Part model, mm, in its own coordinate system. Face numbers are marked on the shaded views. A direction names the side the tool comes from. Coordinates: 2 decimals unless noted, no trailing zeros. Loops run counter-clockwise (first coordinate to the right, second up) from the corner with the lowest first, then second, coordinate; pieces in that order, holes last. Notation, with made-up numbers: (16.25, 32.25) - (38.25, 32.25) arc R12 ccw to (38.25, 38.25) - close; hole circle Ø5 at (-1.75, 25.25). An arc over 180 degrees is marked (long way). Answer as CSV lines item,"result".
from build123d import *

# Parameters (mm, degrees)
SKETCH_1_W          = 4
SKETCH_1_H          = 5.1
EXTRUDE_1_DEPTH     = 5
SKETCH_2_R          = 3
CUT_EXTRUDE_1_DEPTH = 10
SKETCH_3_R          = 7
SKETCH_3_R_2        = 4
EXTRUDE_2_DEPTH     = 4
CHAMFER_1_SIZE      = 0.5
SKETCH_4_R          = 4
CUT_EXTRUDE_2_DEPTH = 10
CUT_EXTRUDE_2_DRAFT = 20


with BuildPart() as part:
    # Эскиз1 → Бобышка-Вытянуть1 (new body)
    with BuildSketch(Plane.XY):
        with BuildLine():
            ThreePointArc((7.674867745, 14.259797906), (4.86875016, 18.350131705), (0.190816738, 20))
            Line((0.190816738, 20), (-0.190816738, 20))
            ThreePointArc((-0.190816738, 20), (-4.86875016, 18.350131705), (-7.674867745, 14.259797906))
            Line((-7.674867745, 14.259797906), (-12.5, 0))
            Line((-12.5, 0), (-12.5, -20))
            Line((-12.5, -20), (12.5, -20))
            Line((12.5, -20), (12.5, 0))
            Line((12.5, 0), (7.674867745, 14.259797906))
        make_face()
        Polygon((15, -32.1), (15, -28.1), (11, -28.1), (-11, -28.1), (-15, -28.1), (-15, -32.1), align=None)
        with Locations((13, -25.55)):
            Rectangle(SKETCH_1_W, SKETCH_1_H)
        Polygon((15, -20), (12.5, -20), (-12.5, -20), (-15, -20), (-15, -23), (-11, -23), (11, -23), (15, -23), align=None)
        with Locations((-13, -25.55)):
            Rectangle(SKETCH_1_W, SKETCH_1_H)
    extrude(amount=EXTRUDE_1_DEPTH)

    # Эскиз2 → Вырез-Вытянуть1 (cut)
    with BuildSketch(Plane.XY.offset(5)):
        with Locations((0, 10)):
            Circle(SKETCH_2_R)
    extrude(amount=-CUT_EXTRUDE_1_DEPTH, mode=Mode.SUBTRACT)

    # Эскиз3 → Бобышка-Вытянуть2 (add)
    with BuildSketch(Plane.XY.offset(5)):
        with Locations((0, -8)):
            Circle(SKETCH_3_R)
        with Locations((0, -8)):
            Circle(SKETCH_3_R_2, mode=Mode.SUBTRACT)
    extrude(amount=EXTRUDE_2_DEPTH)

    # Фаска1
    chamfer_1_edges = [part.edges().sort_by_distance(p)[0] for p in [
        (-7, -8, 9),
    ]]
    chamfer(chamfer_1_edges, length=CHAMFER_1_SIZE)


with BuildPart() as cut_extrude_2_tool:
    # Эскиз4 → Вырез-Вытянуть2 (with draft: the straight prism first)
    with BuildSketch(Plane.XY.offset(5)):
        with Locations((0, -8)):
            Circle(SKETCH_4_R)
    extrude(amount=-CUT_EXTRUDE_2_DEPTH)
    # Вырез-Вытянуть2: the draft: its side faces are tilted about the plane it starts from
    cut_extrude_2_sides = [cut_extrude_2_tool.faces().sort_by_distance(p)[0] for p in [
        (-4, -8, 0),
    ]]
    draft(cut_extrude_2_sides, Plane.XY.offset(5), CUT_EXTRUDE_2_DRAFT)


with BuildPart() as part_1:
    add(part.part)

    # Вырез-Вытянуть2: cut by cut_extrude_2_tool
    add(cut_extrude_2_tool.part, mode=Mode.SUBTRACT)


solid = part_1.part
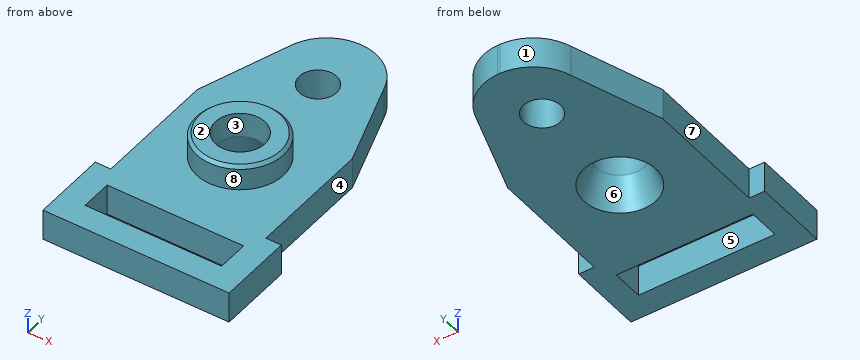
Q1. Two-plate mould, pull along X, no slides. Class the marked faces 1, 2 and 3: released by +X, released by -X, zero draft, split by the parting line, or undercut.
Results:
face 1,"released by -X"
face 2,"zero draft"
face 3,"undercut"
Q2. Which spindle directions (+Z, -Z, +X, -X, +Y, -Y) get a long thin tool onto all of the face, cutting with end or side? Do the marked faces 4, 5, 6, 7 and 8. Say none if no direction does.
Results:
face 4,"+Z, -Z, +X, +Y"
face 5,"+Z, -Z"
face 6,"-Z"
face 7,"+Z, -Z, -X, +Y"
face 8,"+Z"
Q3. Flat gauge pins, fed straight in: pin 1 (2 mm diameter, centred on x = 4, z = 7, fed in from +Y); pin 2 (5 mm diameter, centred on y = -14.5, z = 6.5, fed in from +X); pin 3 (0.8 mm diameter, centred on x = 14, z = 2.5, fed in from +Y). Where does each tip first touch, or does it go through?
Results:
pin 1,"stops at y = -1.68"
pin 2,"stops at x = 12.5"
pin 3,"stops at y = -20"
Q4. Saw through at D-D (z = 5.5). Give the cut face in (x, y), then the cut area to 3 significant figures.
Results:
outline,"circle Ø14 at (0, -8); hole circle Ø8 at (0, -8)"
area,"104 mm^2"
Q5. Wall check: L1, parallel to X at y = -11, z = 2.25; L2, parallel to Y at x = 0, z = 6.45; L3, parallel to Y at x = 0, z = 1.1. Give the ranges that are in metal, low to high.
Results:
L1,"x = -12.5 to -4, 4 to 12.5"
L2,"y = -15 to -12, -4 to -1"
L3,"y = -32.1 to -28.1, -23 to -13.42, -2.58 to 7, 13 to 20"
Q6. Saw through at A-A (y = -8). Give the cut face in (x, z).
Results:
outline,"(-12.5, 0) - (-5.82, 0) - (-4, 5) - (-4, 9) - (-6.5, 9) - (-7, 8.5) - (-7, 5) - (-12.5, 5) - close; (4, 5) - (5.82, 0) - (12.5, 0) - (12.5, 5) - (7, 5) - (7, 8.5) - (6.5, 9) - (4, 9) - close"
Q7. Saw through at C-C (y = 10). Give the cut face in (x, z).
Results:
outline,"(-9.12, 0) - (-3, 0) - (-3, 5) - (-9.12, 5) - close; (3, 0) - (9.12, 0) - (9.12, 5) - (3, 5) - close"
Q8. Saw through at B-B (z = 1.75). Give the cut face in (x, y), then the cut area to 3 significant figures.
Results:
outline,"(-15, -32.1) - (15, -32.1) - (15, -20) - (12.5, -20) - (12.5, 0) - (7.67, 14.26) arc R8 ccw to (0.19, 20) - (-0.19, 20) arc R8 ccw to (-7.67, 14.26) - (-12.5, 0) - (-12.5, -20) - (-15, -20) - close; hole (-11, -28.1) - (11, -28.1) - (11, -23) - (-11, -23) - close; hole circle Ø10.37 at (0, -8); hole circle Ø6 at (0, 10)"
area,"991 mm^2"
